Check sheet for the modelled part. Datum: model origin and axes. Units: mm. Face numbers are marked on the shaded views. Coordinates: 2 decimals unless noted, no trailing zeros. Write each loop counter-clockwise with the first axis right and the second up, starting at its lowest first coordinate (ties: lowest second). Pieces come first, ordered by that corner, then holes. Notation, with made-up numbers: M -8.5,-31 L 37.5,-31 A19 cw 37.5,-19 Z; hole C 3.25,79 d11. An arc over 180 degrees is marked long. Answer as CSV lines item,"result". Start each with the question number.
Q1. Mould release check, pull along Y, two halves, no side actions. Record for the marked faces 1, 2 and 3: pulls with the +Y half, pulls with the -Y half, needs draft (parallel to the pull), parting line crosses it, or undercut.
Q2. Sectioned sample at C-C, the plane y = 44.5. Record the cut outline in (x, z).
Q3. Depth check by flat-ended pin: pin 1 Ø4 at (y, z) = (43.5, 18.5) entering from +X; pin 2 Ø4 at (y, z) = (33, 18.5) entering from -X; pin 3 Ø5.5 at (x, z) = (26, 17) entering from -Y; pin 4 Ø12 at (x, y) = (6, 3.5) entering from -Z. Enter the tip coordinate at first touch or a pass-through.
Q4. Thickness scan on line 1 along Y through (x, z) = (0, 8.75); line 2 along Y through (x, z) = (0, 18.05); line 3 along X through (y, z) = (-6, 8.75). Record the ranges inside material, lowest first. Write a range as from..to.
Q5. Sectioned sample at A-A, the plane z = 17.25. Count the separate pieces of the cut face and the enclosed holes in it, then the cut area to 3 significant figures.
Q6. Sectioned sample at D-D, the plane x = 0. Record the cut outline in (y, z), then the cut area to 3 significant figures.
Q7. Sectioned sample at B-B, the plane x = -53.5. Record the cut outline in (y, z), then the cut area to 3 significant figures.
from build123d import *

# Parameters (mm, degrees)
SKETCH2_R           = 65
BOSS_EXTRUDE1_DEPTH = 20
SKETCH3_R           = 58.5
CUT_EXTRUDE1_DEPTH  = 20
SKETCH4_R           = 60.5
SKETCH4_R_2         = 60
CUT_EXTRUDE3_DEPTH  = 5
SKETCH5_R           = 10
BOSS_EXTRUDE2_DEPTH = 20
SKETCH6_R           = 58.5
SKETCH6_R_2         = 10.5
BOSS_EXTRUDE3_DEPTH = 5
CUT_EXTRUDE4_DEPTH  = 5
SKETCH9_R           = 12.5
SKETCH9_R_2         = 10
BOSS_EXTRUDE4_DEPTH = 15


with BuildPart() as part:
    # Sketch2 → Boss-Extrude1 (new body)
    with BuildSketch(Plane.XY):
        Circle(SKETCH2_R)
    extrude(amount=BOSS_EXTRUDE1_DEPTH)

    # Sketch3 → Cut-Extrude1 (cut)
    with BuildSketch(Plane.XY.offset(20)):
        Circle(SKETCH3_R)
    extrude(amount=-CUT_EXTRUDE1_DEPTH, mode=Mode.SUBTRACT)

    # Sketch4 → Cut-Extrude3 (cut)
    with BuildSketch(Plane.XY.offset(20)):
        Circle(SKETCH4_R)
        Circle(SKETCH4_R_2, mode=Mode.SUBTRACT)
    extrude(amount=-CUT_EXTRUDE3_DEPTH, mode=Mode.SUBTRACT)

    # Sketch6 → Boss-Extrude3 (add)
    with BuildSketch(Plane.XY.offset(20)):
        Circle(SKETCH6_R)
        Circle(SKETCH6_R_2, mode=Mode.SUBTRACT)
    extrude(amount=-BOSS_EXTRUDE3_DEPTH)

    # Sketch8 → Cut-Extrude4 (cut)
    with BuildSketch(Plane.XY.offset(20)):
        with BuildLine():
            Line((-2.5, 12.247448714), (-2.5, 55.5))
            ThreePointArc((-2.5, 55.5), (-39.284220751, 39.284220751), (-55.5, 2.5))
            Line((-55.5, 2.5), (-12.247448714, 2.5))
            ThreePointArc((-12.247448714, 2.5), (-8.838834765, 8.838834765), (-2.5, 12.247448714))
        make_face()
        with BuildLine():
            Line((2.5, -12.247448714), (2.5, -55.5))
            ThreePointArc((2.5, -55.5), (39.284220751, -39.284220751), (55.5, -2.5))
            Line((55.5, -2.5), (12.247448714, -2.5))
            ThreePointArc((12.247448714, -2.5), (8.838834765, -8.838834765), (2.5, -12.247448714))
        make_face()
        with BuildLine():
            Line((12.247448714, 2.5), (55.5, 2.5))
            ThreePointArc((55.5, 2.5), (39.284220751, 39.284220751), (2.5, 55.5))
            Line((2.5, 55.5), (2.5, 12.247448714))
            ThreePointArc((2.5, 12.247448714), (8.838834765, 8.838834765), (12.247448714, 2.5))
        make_face()
        with BuildLine():
            ThreePointArc((-12.247448714, -2.5), (-8.838834765, -8.838834765), (-2.5, -12.247448714))
            Line((-2.5, -12.247448714), (-2.5, -55.5))
            ThreePointArc((-2.5, -55.5), (-39.284220751, -39.284220751), (-55.5, -2.5))
            Line((-55.5, -2.5), (-12.247448714, -2.5))
        make_face()
    extrude(amount=-CUT_EXTRUDE4_DEPTH, mode=Mode.SUBTRACT)



with BuildPart() as body_2:
    # Sketch5 → Boss-Extrude2 (new body)
    with BuildSketch(Plane.XY.offset(20)):
        Circle(SKETCH5_R)
    extrude(amount=-BOSS_EXTRUDE2_DEPTH)


with BuildPart() as part_1:
    add(part.part)

    add(body_2.part)  # Boss-Extrude4 merges body 2
    # Sketch9 → Boss-Extrude4 (add)
    with BuildSketch(Plane(origin=(0, 0, 15), x_dir=(-1, 0, 0), z_dir=(0, 0, -1))):
        Circle(SKETCH9_R)
        Circle(SKETCH9_R_2, mode=Mode.SUBTRACT)
    extrude(amount=BOSS_EXTRUDE4_DEPTH)


solid = part_1.part
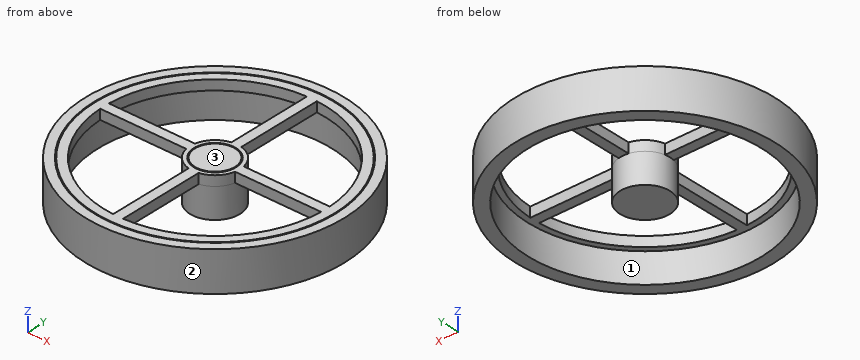
Output:
1,face 1,"undercut"
1,face 2,"parting line crosses it"
1,face 3,"needs draft"
2,outline,"M -47.38,0 L -37.97,0 L -37.97,15 L -33.26,15 L -33.26,20 L -40.25,20 L -40.25,15 L -40.99,15 L -40.99,20 L -47.38,20 Z; M -2.5,15 L 2.5,15 L 2.5,20 L -2.5,20 Z; M 33.26,15 L 37.97,15 L 37.97,0 L 47.38,0 L 47.38,20 L 40.99,20 L 40.99,15 L 40.25,15 L 40.25,20 L 33.26,20 Z"
3,pin 1,"stops at x = 50.03"
3,pin 2,"stops at x = -57.13"
3,pin 3,"stops at y = -60.7"
3,pin 4,"stops at z = 0"
4,line 1,"y = -65..-58.5, -12.5..12.5, 58.5..65"
4,line 2,"y = -65..-60.5, -60..-10.5, -10..10, 10.5..60, 60.5..65"
4,line 3,"x = -64.72..-58.19, -10.97..10.97, 58.19..64.72"
5,separate pieces,"3"
5,enclosed holes,"6"
5,area,"4,710 mm^2"
6,outline,"M -65,0 L -58.5,0 L -58.5,15 L -12.5,15 L -12.5,0 L 12.5,0 L 12.5,15 L 58.5,15 L 58.5,0 L 65,0 L 65,20 L 60.5,20 L 60.5,15 L 60,15 L 60,20 L 10.5,20 L 10.5,15 L 10,15 L 10,20 L -10,20 L -10,15 L -10.5,15 L -10.5,20 L -60,20 L -60,15 L -60.5,15 L -60.5,20 L -65,20 Z"
6,area,"1,210 mm^2"
7,outline,"M -36.92,0 L -23.66,0 L -23.66,15 L -14.97,15 L -14.97,20 L -27.16,20 L -27.16,15 L -28.25,15 L -28.25,20 L -36.92,20 Z; M -2.5,15 L 2.5,15 L 2.5,20 L -2.5,20 Z; M 14.97,15 L 23.66,15 L 23.66,0 L 36.92,0 L 36.92,20 L 28.25,20 L 28.25,15 L 27.16,15 L 27.16,20 L 14.97,20 Z"
7,area,"631 mm^2"
